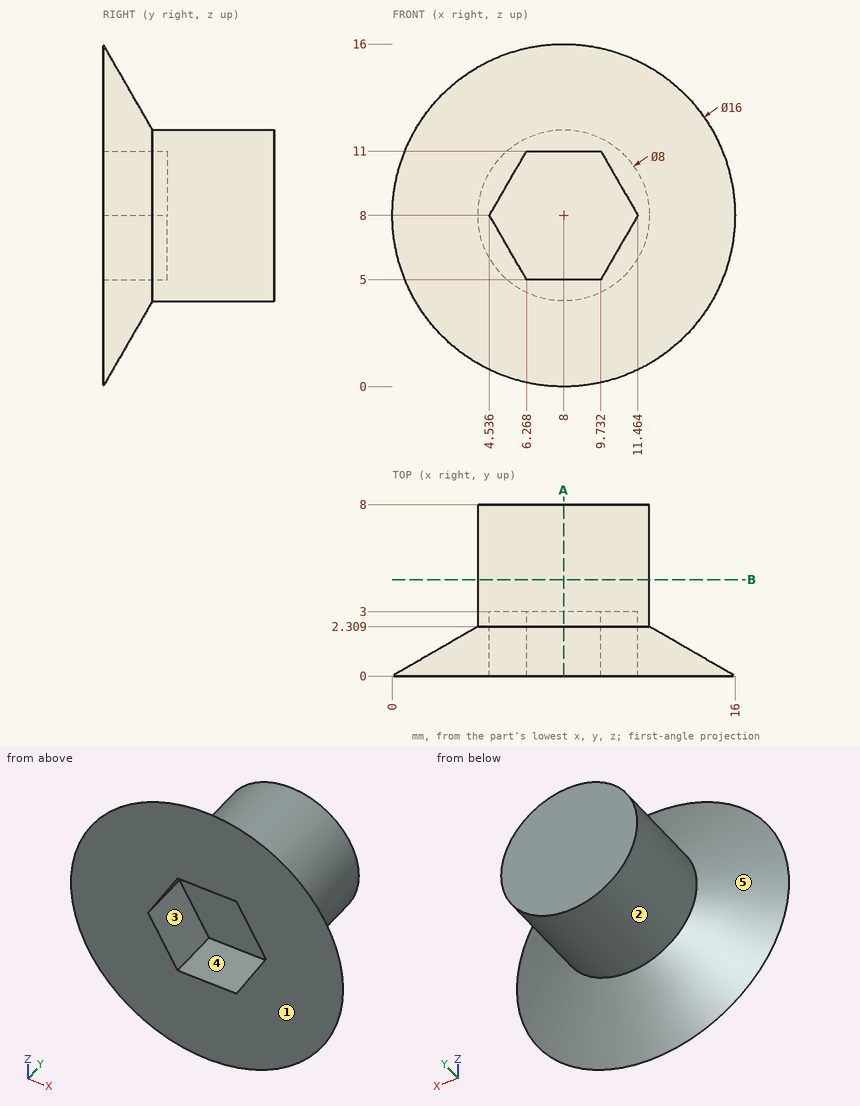
Study the drawing (mm; zero at the part's minimum x, y, z) and answer. A direction names the side the tool comes from. Give positions to 0.01 mm unless a question says otherwise; leave off trailing zeros. Order: outer loops, then holes, each group sorted by start corner. A loop starts at its lowest first (then second) coordinate and runs counter-clockwise, first axis right, second up. Notation, with made-up numbers: (28.5, 12.5) - (79.5, 12.5) arc R13 ccw to (79.5, 16.5) - close; hole circle Ø8 at (16.25, 61). An arc over 180 degrees is marked (long way). Answer as CSV lines item,"result". Start each with the question number.
Q1. Find the intervals of material crossed by L1, parallel to X at y = 2, z = 6.75 (1 decimal); L2, parallel to X at y = 2.25, z = 8.5 (1 decimal); L3, parallel to Z at x = 8, y = 2.25 (1 decimal), in increasing order. Write a range as [from, to].
Q2. The part is cut by section A-A (x = 8). Write down the section's boundary in (y, z).
Q3. The mould has two halves that part along Z. Classify the marked faces 1, 2 and 3: +Z half, -Z half, draft (parallel to the pull), parting line (faces both ways), or undercut.
Q4. The part is cut by section B-B (y = 4.5). Write down the section's boundary in (x, z).
Q5. For the marked faces 4 and 5, determine the directions among +Z, -Z, +X, -X, +Y, -Y from which every point of the face is accessible in a straight line to the end or side of a thin tool.
Q6. Given pin 1 Ø2.5 at (x, y) = (8.5, 2) entering from -Z (1 decimal); pin 2 Ø2 at (x, z) = (9, 12.5) entering from -Y; pin 3 Ø2.5 at (x, y) = (8, 2) entering from +Z, each flat-ended and moving along its own axis, determine where each tip first touches the part or whether it passes through.
Check result:
1,L1,"x = [3.6, 5.3], [10.7, 12.4]"
1,L2,"x = [3.9, 4.8], [11.2, 12.1]"
1,L3,"z = [3.9, 5], [11, 12.1]"
2,outline,"(0, 0) - (2.31, 4) - (8, 4) - (8, 12) - (2.31, 12) - (0, 16) - (0, 11) - (3, 11) - (3, 5) - (0, 5) - close"
3,face 1,"draft"
3,face 2,"parting line"
3,face 3,"undercut"
4,outline,"circle Ø8 at (8, 8)"
5,face 4,"-Y"
5,face 5,"+Y"
6,pin 1,"stops at z = 1.3"
6,pin 2,"stops at y = 0"
6,pin 3,"stops at z = 14.7"
